from build123d import *

# Parameters (mm, degrees)
SKETCH7_W           = 10.005786465
SKETCH7_H           = 9.409830531
BOSS_EXTRUDE2_DEPTH = 12.7
SKETCH8_R           = 2.9718
CUT_EXTRUDE1_DEPTH  = 5.588
CUT_EXTRUDE1_TAPER  = 1.05
SKETCH11_R          = 2.869383086
CUT_EXTRUDE2_DEPTH  = 8.112


with BuildPart() as part:
    # Sketch7 → Boss-Extrude2 (new body)
    with BuildSketch(Plane(origin=(0, 0, 0), x_dir=(1, 0, 0), z_dir=(0, 1, 0))):
        with Locations((-0.145137292, 0.156830508)):
            Rectangle(SKETCH7_W, SKETCH7_H)
    extrude(amount=BOSS_EXTRUDE2_DEPTH)

    # Sketch8 → Cut-Extrude1 (cut)
    with BuildSketch(Plane(origin=(0, 12.7, 0), x_dir=(1, 0, 0), z_dir=(0, 1, 0))):
        Circle(SKETCH8_R)
    extrude(amount=-CUT_EXTRUDE1_DEPTH, taper=CUT_EXTRUDE1_TAPER, mode=Mode.SUBTRACT)

    # Sketch11 → Cut-Extrude2 (cut, through all)
    with BuildSketch(Plane(origin=(0, 7.112, 0), x_dir=(1, 0, 0), z_dir=(0, 1, 0))):
        Circle(SKETCH11_R)
    extrude(amount=-CUT_EXTRUDE2_DEPTH, mode=Mode.SUBTRACT)


solid = part.part
The listing builds one solid part. Answer for the finished solid, in the listing's coordinates (mm). Round coordinates to 2 decimals unless told otherwise and drop trailing zeros. Write each loop counter-clockwise with the first axis right and the second up, starting at its lowest first coordinate (ties: lowest second). Pieces come first, ordered by that corner, then holes. Notation, with made-up numbers: M 6,17 L 42,17 A21 ccw 42,54 Z; hole C 15,18.25 d7. An arc over 180 degrees is marked long. Write each question's results on one line, items separated by ' | '. Start each with the question number.
Item 1: The mould has two halves that part along X. Classify faces 1 (the flat face through (-5.148, 6, 0)), 2 (the cylindrical face through (-0.62, 3.61, 2.8)), 3 (the conical face through (2.785, 9.867, -0.877)), 4 (the flat face through (0, 6, -4.862)): +X half, -X half, draft (parallel to the pull), parting line (faces both ways), or undercut.
Item 2: Find section A-A on y = 4.25. Write down the section's boundary in (x, z), and give its area (3 significant figures).
Item 3: Straight lines are drawn through the part: probe 1 along X at (y, z) = (4.5, 0); probe 2 along Z at (x, y) = (0, 4.75); probe 3 along X at (y, z) = (10.5, -2). For each, find the intervals that lie inside material, in ascending order.
Answer block:
1) face 1: -X half | face 2: undercut | face 3: undercut | face 4: draft
2) outline: M -5.15,-4.86 L 4.86,-4.86 L 4.86,4.55 L -5.15,4.55 Z; hole C 0,0 d5.74 | area: 68.3 mm²
3) probe 1: x = -5.15 to -2.87, 2.87 to 4.86 | probe 2: z = -4.86 to -2.87, 2.87 to 4.55 | probe 3: x = -5.15 to -2.14, 2.14 to 4.86
